Geometry check sheet. Reference: the model listing, model coordinates, mm. Face numbers are marked on the shaded views. A direction names the side the tool comes from. Round coordinates to 2 decimals unless told otherwise and drop trailing zeros. Order: outer loops, then holes, each group sorted by start corner. A loop starts at its lowest first (then second) coordinate and runs counter-clockwise, first axis right, second up.
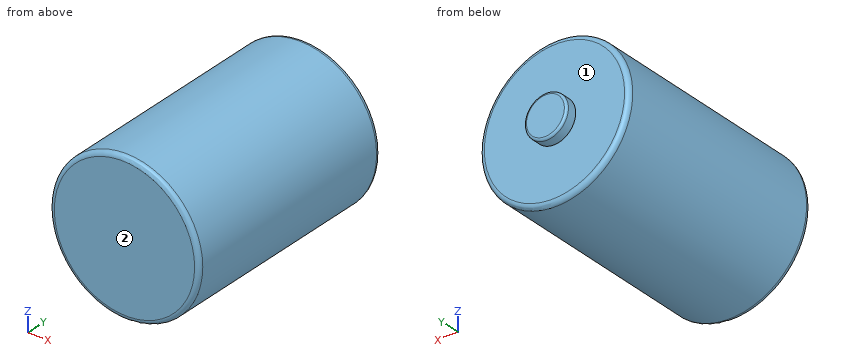
```python
from build123d import *

# Parameters (mm, degrees)
F0_R     = 41.81566
F1_DEPTH = 127
F2_R     = 11.875081
F3_DEPTH = 6.35
F4_R     = 2.54
F5_R     = 2.54
F6_R     = 1.27


with BuildPart() as f1:
    # F0 (on Front) → F1 (new body)
    with BuildSketch(Plane.XZ):
        Circle(F0_R)
    extrude(amount=F1_DEPTH)

    # F2 (on face) → F3 (join)
    with BuildSketch(Plane(origin=(0, 0, 0), x_dir=(-1, 0, 0), z_dir=(0, 1, 0))):
        Circle(F2_R)
    extrude(amount=F3_DEPTH)

    # F4
    f4_edges = [f1.edges().sort_by_distance(p)[0] for p in [
        (-41.81566, 0, 0),
    ]]
    fillet(f4_edges, radius=F4_R)

    # F5
    f5_edges = [f1.edges().sort_by_distance(p)[0] for p in [
        (-41.81566, -127, 0),
    ]]
    fillet(f5_edges, radius=F5_R)

    # F6
    f6_edges = [f1.edges().sort_by_distance(p)[0] for p in [
        (11.875081, 6.35, 0),
    ]]
    fillet(f6_edges, radius=F6_R)


solid = f1.part
```
(1) Sectioned sample at A-A, the plane x = 0. Record the cut outline in (y, z), and give its area (3 significant figures).
Returned:
outline: (-127, -39.28) arc R2.54 ccw to (-124.46, -41.82) - (-2.54, -41.82) arc R2.54 ccw to (0, -39.28) - (0, -11.88) - (5.08, -11.88) arc R1.27 ccw to (6.35, -10.61) - (6.35, 10.61) arc R1.27 ccw to (5.08, 11.88) - (0, 11.88) - (0, 39.28) arc R2.54 ccw to (-2.54, 41.82) - (-124.46, 41.82) arc R2.54 ccw to (-127, 39.28) - close
area: 10,800 mm2
(2) Material ranges on line 1 (Y direction, x = 12, z = -37); line 2 (Z direction, x = 0, y = -6); line 3 (X direction, y = -114.5, z = 1.5), recorded low to high.
Returned:
line 1: y = -127 to 0
line 2: z = -41.82 to 41.82
line 3: x = -41.79 to 41.79
(3) Set-up check for the marked faces 1 and 2: record each of +Z, -Z, +X, -X, +Y, -Y from which the full face is reachable in a straight line by a thin tool's end or side.
Returned:
face 1: +Y
face 2: +Z, -Z, +X, -X, -Y
(4) Sectioned sample at B-B, the plane z = 0. Record the cut outline in (x, y), and give its area (3 significant figures).
Returned:
outline: (-41.82, -124.46) arc R2.54 ccw to (-39.28, -127) - (39.28, -127) arc R2.54 ccw to (41.82, -124.46) - (41.82, -2.54) arc R2.54 ccw to (39.28, 0) - (11.88, 0) - (11.88, 5.08) arc R1.27 ccw to (10.61, 6.35) - (-10.61, 6.35) arc R1.27 ccw to (-11.88, 5.08) - (-11.88, 0) - (-39.28, 0) arc R2.54 ccw to (-41.82, -2.54) - close
area: 10,800 mm2
(5) Depth check by flat-ended pin: P1, Ø2, axis at y = -111, z = 14.5, coming from the +X side; P2, Ø3, axis at y = -27.5, z = -28, coming from the +X side; P3, Ø6, axis at y = -8, z = 7.5, coming from the -X side. Enter the tip coordinate at first touch or a pass-through.
Returned:
P1: stops at x = 39.58
P2: stops at x = 32.35
P3: stops at x = -41.57
(6) Sectioned sample at C-C, the plane y = -85. Record the cut outline in (x, z).
Returned:
outline: circle Ø83.63 at (0, 0)
